For this review, use the dimensioned drawing (mm, ordinates from the lowest corner) and the shaded views. A direction names the side the tool comes from. Round coordinates to 2 decimals unless told otherwise and drop trailing zeros. Order: outer loops, then holes, each group sorted by start corner. A loop starts at its lowest first (then second) coordinate and runs counter-clockwise, first axis right, second up. Notation, with made-up numbers: (16.5, 39) - (73.5, 39) arc R27 ccw to (73.5, 56) - close; hole circle Ø6 at (65.25, 60). An arc over 180 degrees is marked (long way). Write item = value, one per line.
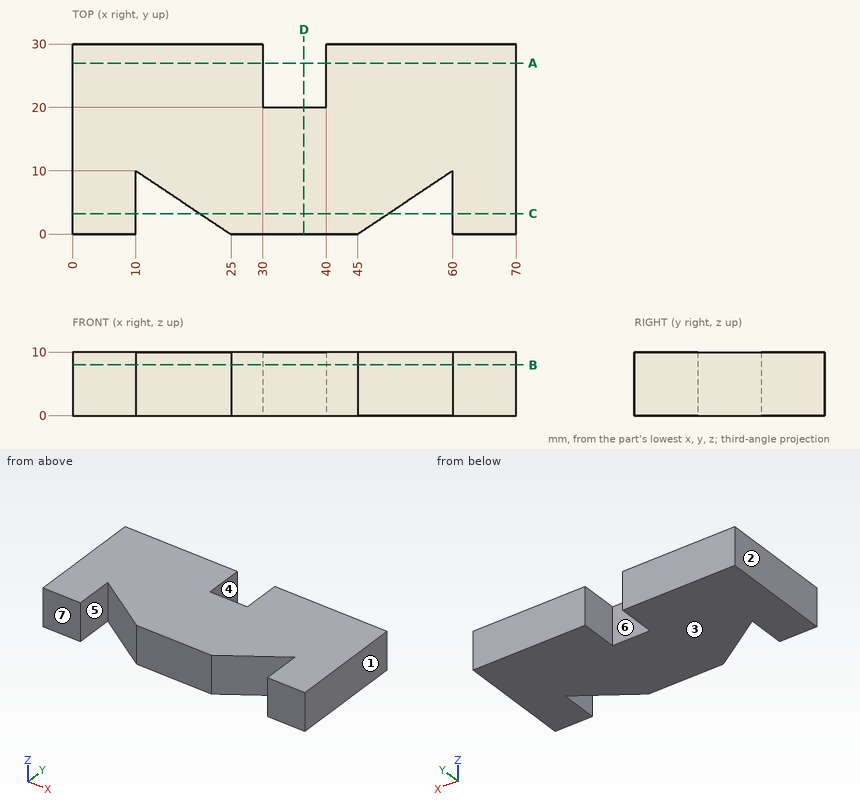
Item 1: The part is to be moulded in two halves that separate along X. For the marked faces 1, 2, 3 and 4, say which applies: +X half, -X half, draft (parallel to the pull), parting line (faces both ways), or undercut.
Data:
face_1 = +X half
face_2 = -X half
face_3 = draft
face_4 = undercut
Item 2: Insertion check: P1, Ø4, axis at x = 48, y = 14, coming from the -Z side. The pin has a flat end and moves straight along its axis. Give the tip position at first contact, or say it passes through.
Data:
P1 = 0
Item 3: Take a section at A-A, the plane y = 27. State the section outline as (x, z) points.
Data:
outline = (0, 0) - (30, 0) - (30, 10) - (0, 10) - close; (40, 0) - (70, 0) - (70, 10) - (40, 10) - close
Item 4: For line 1 along X through (y, z) = (24.25, 9); line 2 along X through (y, z) = (8.25, 7.5) (3 decimals); line 3 along X through (y, z) = (9, 6.5), list the stretches that pass through material, from the lowest coordinate up. Write a range as [from, to].
Data:
line_1 = [0, 30], [40, 70]
line_2 = [0, 10], [12.625, 57.375], [60, 70]
line_3 = [0, 10], [11.5, 58.5], [60, 70]
Item 5: Take a section at B-B, the plane z = 8. State the section outline as (x, y) points, and give its area (3 significant figures).
Data:
outline = (0, 0) - (10, 0) - (10, 10) - (25, 0) - (45, 0) - (60, 10) - (60, 0) - (70, 0) - (70, 30) - (40, 30) - (40, 20) - (30, 20) - (30, 30) - (0, 30) - close
area = 1,850 mm2
Item 6: Take a section at C-C, the plane y = 3.25. State the section outline as (x, z) points (3 decimals).
Data:
outline = (0, 0) - (10, 0) - (10, 10) - (0, 10) - close; (20.125, 0) - (49.875, 0) - (49.875, 10) - (20.125, 10) - close; (60, 0) - (70, 0) - (70, 10) - (60, 10) - close
Item 7: Take a section at D-D, the plane x = 36.5. State the section outline as (y, z) points, and give its area (3 significant figures).
Data:
outline = (0, 0) - (20, 0) - (20, 10) - (0, 10) - close
area = 200 mm2
Item 8: For the marked faces 5, 6 and 7, list the 3-axis set-ups (+Z, -Z, +X, -X, +Y, -Y) from which the entire face can be reached by the end or side of a thin tool; tool diameter is ignored.
Data:
face_5 = +Z, -Z, -Y
face_6 = +Z, -Z, +Y
face_7 = +Z, -Z, +X, -X, -Y
